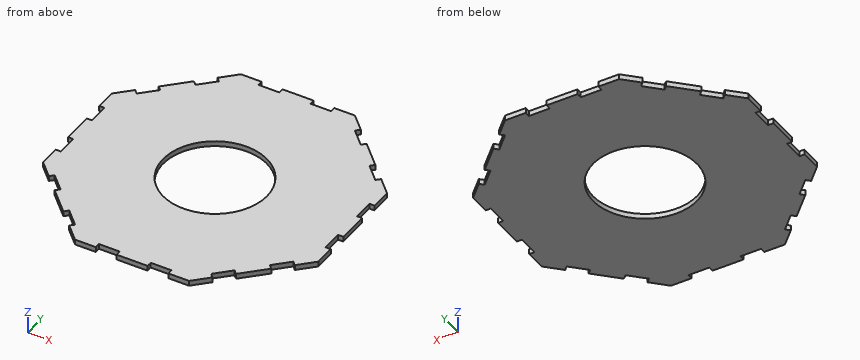
from build123d import *

# Parameters (mm, degrees)
SKETCH1_R           = 31.75
BOSS_EXTRUDE1_DEPTH = 3.175


with BuildPart() as part:
    # Sketch1 → Boss-Extrude1 (new body)
    with BuildSketch(Plane.XY):
        Polygon((41.660192091, 73.091088515), (43.905256121, 75.336152545), (34.925, 84.316408666), (22.225, 84.316408666), (22.225, 81.141408666), (9.525, 81.141408666), (9.525, 84.316408666), (-9.525, 84.316408666), (-9.525, 81.141408666), (-22.225, 81.141408666), (-22.225, 84.316408666), (-34.925, 84.316408666), (-43.905256121, 75.336152545), (-41.660192091, 73.091088515), (-50.640448212, 64.110832393), (-52.885512242, 66.355896424), (-66.355896424, 52.885512242), (-64.110832393, 50.640448212), (-73.091088515, 41.660192091), (-75.336152545, 43.905256121), (-84.316408666, 34.925), (-84.316408666, 22.225), (-81.141408666, 22.225), (-81.141408666, 9.525), (-84.316408666, 9.525), (-84.316408666, -9.525), (-81.141408666, -9.525), (-81.141408666, -22.225), (-84.316408666, -22.225), (-84.316408666, -34.925), (-75.336152545, -43.905256121), (-73.091088515, -41.660192091), (-64.110832393, -50.640448212), (-66.355896424, -52.885512242), (-52.885512242, -66.355896424), (-50.640448212, -64.110832393), (-41.660192091, -73.091088515), (-43.905256121, -75.336152545), (-34.925, -84.316408666), (-22.225, -84.316408666), (-22.225, -81.141408666), (-9.525, -81.141408666), (-9.525, -84.316408666), (9.525, -84.316408666), (9.525, -81.141408666), (22.225, -81.141408666), (22.225, -84.316408666), (34.925, -84.316408666), (43.905256121, -75.336152545), (41.660192091, -73.091088515), (50.640448212, -64.110832393), (52.885512242, -66.355896424), (66.355896424, -52.885512242), (64.110832393, -50.640448212), (73.091088515, -41.660192091), (75.336152545, -43.905256121), (84.316408666, -34.925), (84.316408666, -22.225), (81.141408666, -22.225), (81.141408666, -9.525), (84.316408666, -9.525), (84.316408666, 9.525), (81.141408666, 9.525), (81.141408666, 22.225), (84.316408666, 22.225), (84.316408666, 34.925), (75.336152545, 43.905256121), (73.091088515, 41.660192091), (64.110832393, 50.640448212), (66.355896424, 52.885512242), (52.885512242, 66.355896424), (50.640448212, 64.110832393), align=None)
        Circle(SKETCH1_R, mode=Mode.SUBTRACT)
    extrude(amount=BOSS_EXTRUDE1_DEPTH)


solid = part.part
Check sheet for the modelled part. Datum: model origin and axes. Units: mm. Round coordinates to 2 decimals unless told otherwise and drop trailing zeros. Order: outer loops, then holes, each group sorted by start corner. A loop starts at its lowest first (then second) coordinate and runs counter-clockwise, first axis right, second up. Notation, with made-up numbers: M 85,22 L 104,22 A14 ccw 104,38 Z; hole C 23,25.5 d8. An arc over 180 degrees is marked long. One line per item, written item: value. Start each with the question number.
1. Section check A-A on y = 0. Enter the section's corners in (x, z) (3 decimals), and give its area (3 significant figures).
2. Scan lines: line 1 along X through (y, z) = (1, 0.1); line 2 along Y through (x, z) = (0, 1.5); line 3 along X through (y, z) = (-29.5, 1.1). Record each from-to range of solid material in increasing order.
3. Gauge pin test, flat ends, axial feed: P1, Ø1.6, axis at y = 83, z = 2, coming from the -X side; P2, Ø1, axis at y = 82, z = 1.5, coming from the +X side; P3, Ø1, axis at x = 60, z = 2.5, coming from the +Y side. Record the tip position at first contact, or that the pin passes through.
Results found:
1. outline: M -84.316,0 L -31.75,0 L -31.75,3.175 L -84.316,3.175 Z; M 31.75,0 L 84.316,0 L 84.316,3.175 L 31.75,3.175 Z
1. area: 334 mm^2
2. line 1: -84.32 to -31.73, 31.73 to 84.32
2. line 2: -84.32 to -31.75, 31.75 to 84.32
2. line 3: -84.32 to -11.74, 11.74 to 84.32
3. P1: x = -37.04
3. P2: x = 37.74
3. P3: y = 59.74
